Input: dimensioned drawing with shaded views. Units: mm. Origin: part minimum x, y, z. A direction names the side the tool comes from. Round coordinates to 2 decimals unless told otherwise and drop trailing zeros. Loops run counter-clockwise (first coordinate to the right, second up) from the corner with the lowest first, then second, coordinate; pieces in that order, holes last. Notation, with made-up numbers: M 75.25,22.5 L 131.25,22.5 A7 ccw 131.25,32.5 Z; hole C 72,-6 d5. An arc over 180 degrees is marked long. Put each result on its own line as item: value. Start each with the question number.
1) Pin query (flat end, axial travel): pin 1 (6 mm diameter, centred on x = 13.5, z = 11, fed in from +Y); pin 2 (4.5 mm diameter, centred on x = 6, z = 8, fed in from -Y). Return the tip coordinate at first contact, or that it passes through.
2) Section A-A on x = 11.5. Output: boundary loops of the cut face in (y, z), plus the area to 3 significant figures.
3) Line query: probe 1 along X at (y, z) = (0.85, 31.5); probe 2 along X at (y, z) = (21.25, 35.5); probe 3 along Y at (x, z) = (1.25, 40.5). Output: solid intervals per line, ascending.
4) Draft query along Z for the marked faces 1, 2 and 3. Return one class per face: +Z half, -Z half, draft (parallel to the pull), parting line (faces both ways), or undercut.
5) Reachability of the marked faces 4, 5 and 6 from +Z, -Z, +X, -X, +Y, -Y: full face, straight path, thin tool, end or side. Return the list, or none.
6) Section D-D on x = 20.25. Output: boundary loops of the cut face in (y, z), plus the area to 4 significant figures.
7) Section B-B on z = 31.5. Output: boundary loops of the cut face in (x, y).
8) Section C-C on y = 8. Output: boundary loops of the cut face in (x, z).
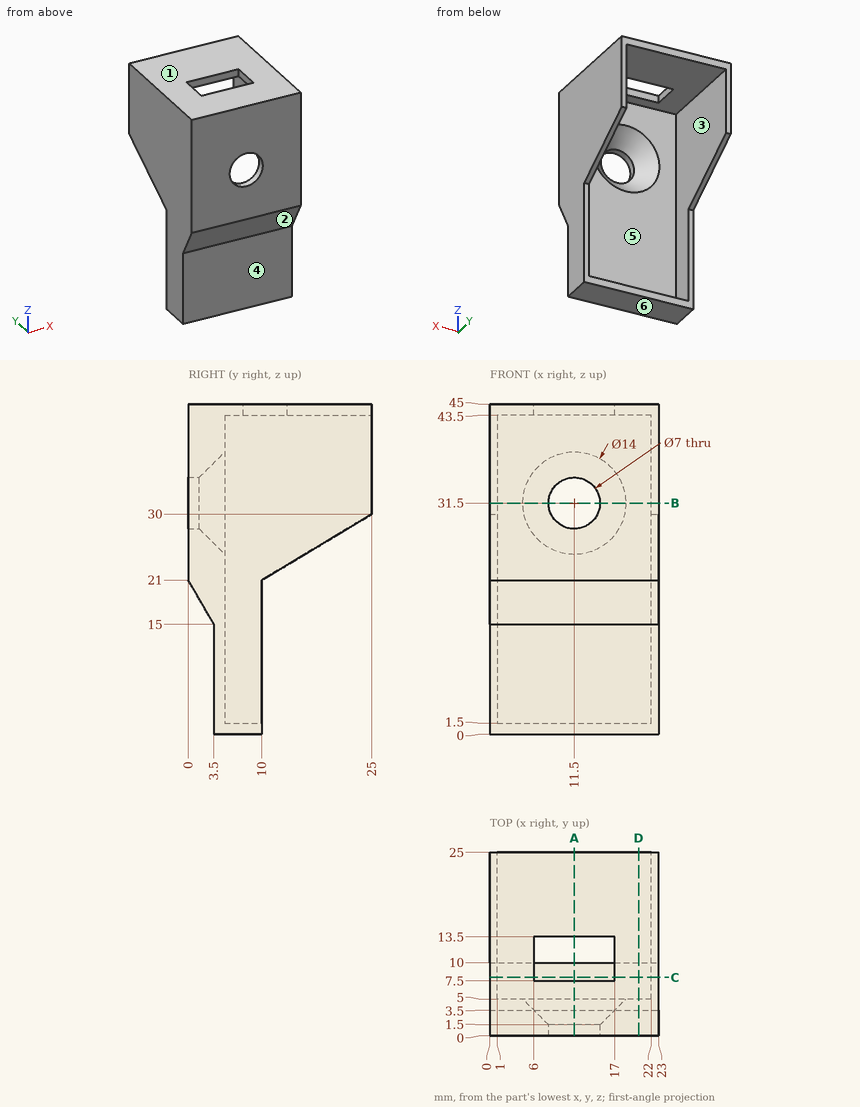
Geometry results:
1. pin 1: stops at y = 5
1. pin 2: stops at y = 3.5
2. outline: M 0,21 L 3.5,15 L 3.5,0 L 10,0 L 10,1.5 L 5,1.5 L 5,24.5 L 1.5,28 L 0,28 Z; M 0,35 L 1.5,35 L 5,38.5 L 5,43.5 L 7.5,43.5 L 7.5,45 L 0,45 Z; M 13.5,43.5 L 25,43.5 L 25,45 L 13.5,45 Z
2. area: 143 mm²
3. probe 1: x = 0 to 8, 15 to 23
3. probe 2: x = 0 to 1, 22 to 23
3. probe 3: y = 0 to 5
4. face 1: +Z half
4. face 2: -Z half
4. face 3: undercut
5. face 4: -Z, +X, -X, -Y
5. face 5: +Y
5. face 6: -Z, +X, -X, +Y, -Y
6. outline: M 0,21 L 3.5,15 L 3.5,0 L 10,0 L 10,1.5 L 5,1.5 L 5,43.5 L 25,43.5 L 25,45 L 0,45 Z
6. area: 199.5 mm²
7. outline: M 0,0 L 8,0 L 8,1.5 L 4.5,5 L 1,5 L 1,25 L 0,25 Z; M 15,0 L 23,0 L 23,25 L 22,25 L 22,5 L 18.5,5 L 15,1.5 Z
8. outline: M 0,0 L 23,0 L 23,45 L 17,45 L 17,43.5 L 22,43.5 L 22,1.5 L 1,1.5 L 1,43.5 L 6,43.5 L 6,45 L 0,45 Z
